The figure shows three views and two pictorial views of one solid part (mm, origin at its lowest corner). Answer the questions. A direction names the side the tool comes from. Round coordinates to 2 decimals unless told otherwise and drop trailing zeros. Order: outer loops, then holes, each group sorted by start corner. A loop starts at its lowest first (then second) coordinate and runs counter-clockwise, first axis right, second up. Notation, with made-up numbers: (-14.5, -22.5) - (36.5, -22.5) arc R26 ccw to (36.5, 8.5) - close; hole circle Ø1 at (37, -28). An arc over 180 degrees is marked (long way). Answer in a Markdown table with one row per item.
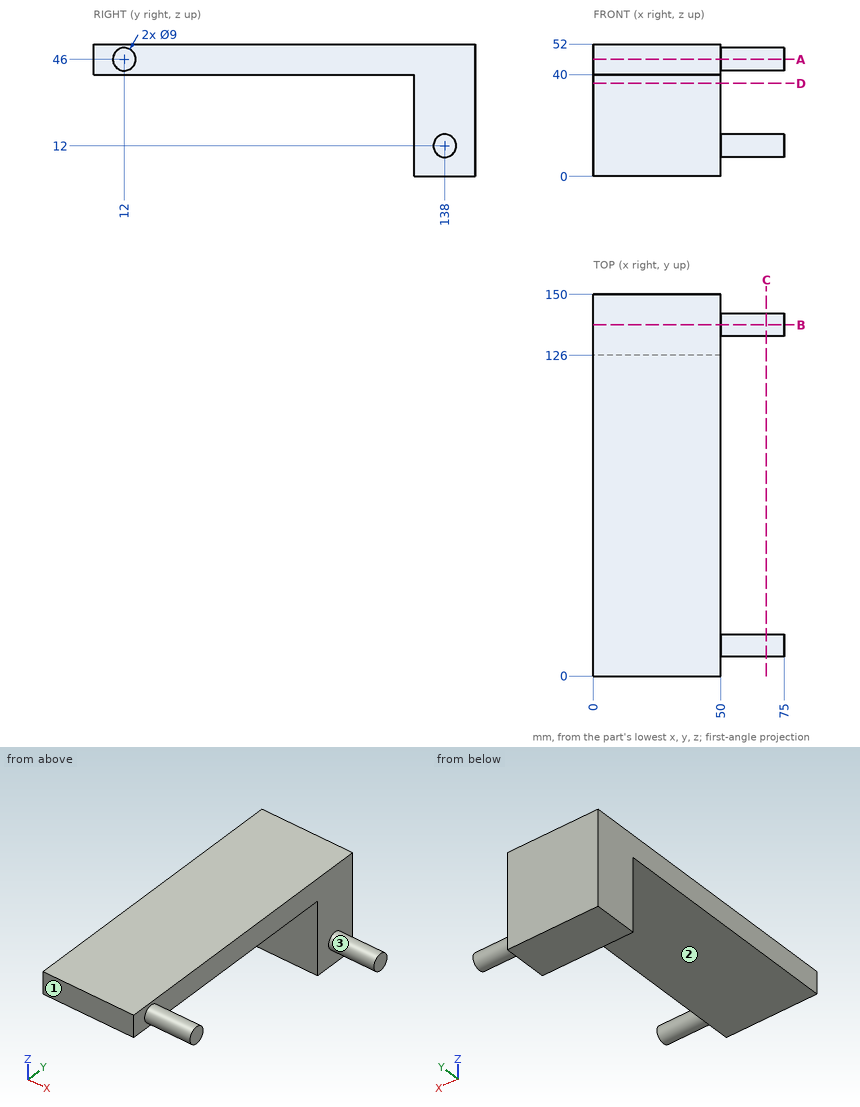
1) Each of these flat-tipped pins is pushed along its axis until it touches: pin 1 (12 mm diameter, centred on x = 25.5, z = 16.5, fed in from -Y); pin 2 (3 mm diameter, centred on x = 60, z = 6.5, fed in from +Y); pin 3 (25 mm diameter, centred on x = 15, y = 44.5, fed in from -Z). Where does it stop, or does it pass through?
Filled in:
| item | result |
|---|---|
| pin 1 | stops at y = 126 |
| pin 2 | stops at y = 140.06 |
| pin 3 | stops at z = 40 |
2) Find section C-C, the plane x = 68. Give the vertices of the cut face in (y, z), then the cut area to 3 significant figures.
Filled in:
| item | result |
|---|---|
| outline | circle Ø9 at (12, 46); circle Ø9 at (138, 12) |
| area | 127 mm^2 |
3) Which of the six approach directions +Z, -Z, +X, -X, +Y, -Y give full straight-line access (tool end or side, diameter ignored) to the marked faces 1, 2 and 3?
Filled in:
| item | result |
|---|---|
| face 1 | +Z, -Z, +X, -X, -Y |
| face 2 | -Z, +X, -X, -Y |
| face 3 | +X |
4) Find section A-A, the plane z = 46. Give the vertices of the cut face in (x, y), then the cut area to 4 significant figures.
Filled in:
| item | result |
|---|---|
| outline | (0, 0) - (50, 0) - (50, 7.5) - (75, 7.5) - (75, 16.5) - (50, 16.5) - (50, 150) - (0, 150) - close |
| area | 7,725 mm^2 |
5) Find the intervals of material crossed by probe 1 along Z at (x, y) = (47, 86); probe 2 along X at (y, z) = (42, 43); probe 3 along Y at (x, z) = (16, 39), in increasing order. Write a range as from..to.
Filled in:
| item | result |
|---|---|
| probe 1 | z = 40..52 |
| probe 2 | x = 0..50 |
| probe 3 | y = 126..150 |
6) Find section D-D, the plane z = 36.5. Give the vertices of the cut face in (x, y), then the cut area to 3 significant figures.
Filled in:
| item | result |
|---|---|
| outline | (0, 126) - (50, 126) - (50, 150) - (0, 150) - close |
| area | 1,200 mm^2 |
7) Find section B-B, the plane y = 138. Give the vertices of the cut face in (x, z), then the cut area to 4 significant figures.
Filled in:
| item | result |
|---|---|
| outline | (0, 0) - (50, 0) - (50, 7.5) - (75, 7.5) - (75, 16.5) - (50, 16.5) - (50, 52) - (0, 52) - close |
| area | 2,825 mm^2 |
